The listing builds one solid part. Answer for the finished solid, in the listing's coordinates (mm). A direction names the side the tool comes from. Coordinates: 2 decimals unless noted, no trailing zeros. Order: outer loops, then holes, each group sorted by start corner. A loop starts at its lowest first (then second) coordinate and runs counter-clockwise, first axis right, second up. Notation, with made-up numbers: (-13, 13) -> (4, 13) arc R19 cw to (4, 33) -> close; hole circle Ø3 at (-14, 7). An arc over 180 degrees is marked (long way). Write each question's results on one line, items separated by ' | '. Start each with the question number.
(1) A tool of negligible diameter and unlimited length cuts with its end or side. For faces 3 (the face through (5, -24, 95)), 4 (the face through (-24, 0, 91)), 5 (the face through (-17, -17, 91)), from which of +Z, -Z, +X, -X, +Y, -Y can it reach the whole face along a straight path? Write none if from no direction.
(2) Determine the mould class of faces 1 (the face through (-24, 5, 95)), 2 (the face through (5, 24, 95)) for opening direction X: +X half, -X half, draft (parallel to the pull), parting line (faces both ways), or undercut.
(3) Straight lines are drawn through the part: L1, parallel to Y at x = 0, z = 88; L2, parallel to Z at x = -2, y = 11.5; L3, parallel to Z at x = 16, y = 21. For each, find the intervals that lie inside material, in ascending order.
(4) Given pin 1 (7 mm diameter, centred on x = -24.5, z = 97.5, fed in from -Y); pin 2 (16.5 mm diameter, centred on x = -20, y = 14.5, fed in from +Z); pin 3 (1 mm diameter, centred on x = 16, y = -3, fed in from +Z); pin 4 (5 mm diameter, centred on x = 1.5, y = -24.5, fed in from +Z), each flat-ended and moving along its own axis, determine where each tip first touches the part or whether it passes through.
(5) The part is cut by section A-A, the plane x = 0. Give the vertices of the cut face in (y, z), then the cut area to 3 significant figures.
(6) The part is cut by section C-C, the plane z = 13. Give the vertices of the cut face in (x, y).
(7) The part is cut by section D-D, the plane y = 14. Give the vertices of the cut face in (x, z).
```python
from build123d import *

# Parameters (mm, degrees)
CYLINDER001_R     = 19
CYLINDER001_DEPTH = 20
BOX_W             = 20
BOX_H             = 10
BOX_DEPTH         = 10
ARRAY_COUNT       = 8
CYLINDER_R        = 30
CYLINDER_DEPTH    = 100


with BuildPart() as cilindre001:
    # Cylinder001 → Cylinder001 (new body)
    with BuildSketch(Plane.XY.offset(80)):
        Circle(CYLINDER001_R)
    extrude(amount=CYLINDER001_DEPTH)


with BuildPart() as array:
    # Box → Box (new body)
    with BuildSketch(Plane(origin=(18, -5, 91), x_dir=(1, 0, 0), z_dir=(0, 0, 1))):
        with Locations((10, 5)):
            Rectangle(BOX_W, BOX_H)
    extrude(amount=BOX_DEPTH)

    # Array: Array ×8 about axis
    array_axis = Axis((0, 0, 0), (0, 0, 1))


with BuildPart() as array_1:
    add(array.part)
    for i in range(1, ARRAY_COUNT):
        add(array.part.rotate(array_axis, i * 360 / ARRAY_COUNT))


with BuildPart() as cut001:
    # Cylinder → Cylinder (new body)
    with BuildSketch(Plane.XY):
        Circle(CYLINDER_R)
    extrude(amount=CYLINDER_DEPTH)

    # Cut: cut Array
    add(array_1.part, mode=Mode.SUBTRACT)

    # Cut001: cut Cilindre001
    add(cilindre001.part, mode=Mode.SUBTRACT)


solid = cut001.part
```
Established:
1) face 3: +Z, +Y, -Y | face 4: +Z, +X, -X | face 5: +Z
2) face 1: draft | face 2: undercut
3) L1: y = -30 to -19, 19 to 30 | L2: z = 0 to 80 | L3: z = 0 to 91
4) pin 1: stops at y = -17.38 | pin 2: stops at z = 100 | pin 3: stops at z = 80 | pin 4: stops at z = 91
5) outline: (-30, 0) -> (30, 0) -> (30, 91) -> (19, 91) -> (19, 80) -> (-19, 80) -> (-19, 91) -> (-30, 91) -> close | area: 5,040 mm^2
6) outline: circle Ø60 at (0, 0)
7) outline: (-26.53, 0) -> (26.53, 0) -> (26.53, 100) -> (21.07, 100) -> (21.07, 91) -> (12.85, 91) -> (12.85, 80) -> (-12.85, 80) -> (-12.85, 91) -> (-21.07, 91) -> (-21.07, 100) -> (-26.53, 100) -> close
